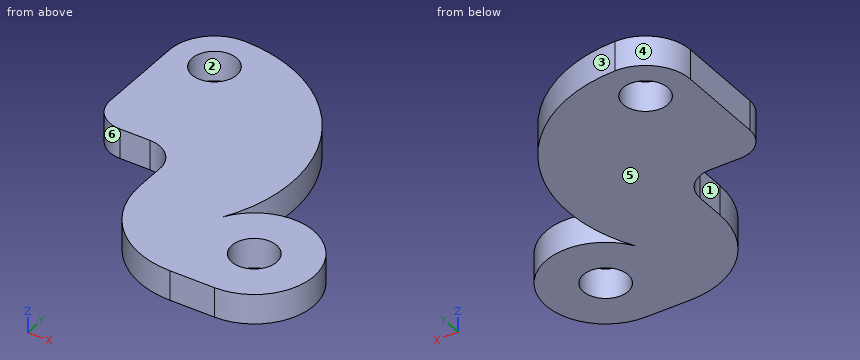
```python
from build123d import *

# Parameters (mm, degrees)
SKETCH1_R           = 7.5
BOSS_EXTRUDE1_DEPTH = 5


with BuildPart() as part:
    # Sketch1 → Boss-Extrude1 (new body, symmetric)
    with BuildSketch(Plane.XY):
        with BuildLine():
            Line((-15, 0), (-15, -30))
            ThreePointArc((-15, -30), (-12.071067812, -37.071067812), (-5, -40))
            Line((-5, -40), (5, -40))
            ThreePointArc((5, -40), (12.071067812, -42.928932188), (15, -50))
            Line((15, -50), (15, -60))
            ThreePointArc((15, -60), (23.786796564, -81.213203436), (45, -90))
            Line((45, -90), (60, -90))
            ThreePointArc((60, -90), (77.320959018, -60.000781096), (42.680393915, -59.998437869))
            ThreePointArc((42.680393915, -59.998437869), (42.903012663, -10.380159149), (0.265123413, 14.997656803))
            ThreePointArc((0.265123413, 14.997656803), (-10.512448545, 10.699926429), (-15, 0))
        make_face()
        Circle(SKETCH1_R, mode=Mode.SUBTRACT)
        with Locations((60, -70)):
            Circle(SKETCH1_R, mode=Mode.SUBTRACT)
    extrude(amount=BOSS_EXTRUDE1_DEPTH, both=True)


solid = part.part
```
The listing builds one solid part. Answer for the finished solid, in the listing's coordinates (mm). Face numbers are marked on the shaded views. A direction names the side the tool comes from. Round coordinates to 2 decimals unless told otherwise and drop trailing zeros. Order: outer loops, then holes, each group sorted by start corner. A loop starts at its lowest first (then second) coordinate and runs counter-clockwise, first axis right, second up. Notation, with made-up numbers: (20, 83) - (77, 83) arc R14 ccw to (77, 95) - close; hole circle Ø4 at (69.25, -10). An arc over 180 degrees is marked (long way). Put each result on its own line as item: value. Start each with the question number.
(1) Find section D-D (y = -25). Give the vertices of the cut face in (x, z), plus the area to 3 significant figures.
(2) Straight lines are drawn through the part: probe 1 along Y at (x, z) = (60, 2); probe 2 along Y at (x, z) = (0, 3.25); probe 3 along X at (y, z) = (-65, -2). For each, find the intervals that lie inside material, in ascending order. Write a range as from..to.
(3) Find section A-A (z = 1.25). Give the vertices of the cut face in (x, y), plus the area to 3 significant figures.
(4) Determine the mould class of the marked faces 3, 4, 5 and 6 for opening direction Y: released by +Y, released by -Y, zero draft, split by the parting line, or undercut.
(5) Given P1, Ø3, axis at x = 59.5, z = -3.5, coming from the +Y side; P2, Ø13.5, axis at x = 0, y = 0, coming from the -Z side; P3, Ø3, axis at y = -57.5, z = -1.5, coming from the -X side; P4, Ø3, axis at x = -2, z = 1, coming from the -Y side, each flat-ended and moving along its own axis, determine where each tip first touches the part or whether it passes through.
(6) Find section B-B (y = -70). Give the vertices of the cut face in (x, z).
(7) Find section C-C (x = 28). Give the vertices of the cut face in (y, z).
(8) For the marked faces 1 and 2, determine the directions among +Z, -Z, +X, -X, +Y, -Y from which every point of the face is accessible in a straight line to the end or side of a thin tool.
Reply:
1. outline: (-15, -5) - (48.37, -5) - (48.37, 5) - (-15, 5) - close
1. area: 634 mm^2
2. probe 1: -90..-77.5, -62.5..-50
2. probe 2: -40..-7.5, 7.5..15
2. probe 3: 15.42..54.41, 65.59..79.36
3. outline: (-15, -30) arc R10 ccw to (-5, -40) - (5, -40) arc R10 cw to (15, -50) - (15, -60) arc R30 ccw to (45, -90) - (60, -90) arc R20 ccw (long way) to (42.68, -60) arc R50 ccw to (0.27, 15) arc R15 ccw to (-15, 0) - close; hole circle Ø15 at (0, 0); hole circle Ø15 at (60, -70)
3. area: 5,140 mm^2
4. face 3: undercut
4. face 4: released by +Y
4. face 5: zero draft
4. face 6: released by -Y
5. P1: y = -50
5. P2: through
5. P3: x = 15
5. P4: y = -40
6. outline: (16.72, -5) - (52.5, -5) - (52.5, 5) - (16.72, 5) - close; (67.5, -5) - (80, -5) - (80, 5) - (67.5, 5) - close
7. outline: (-84.72, -5) - (6.01, -5) - (6.01, 5) - (-84.72, 5) - close
8. face 1: +Z, -Z, -X, -Y
8. face 2: +Z, -Z
